Build history of the part. All positions in model axes, mm. A direction names the side the tool comes from. Give positions to 0.01 mm unless a question says otherwise; leave off trailing zeros. Write each loop counter-clockwise with the first axis right and the second up, starting at its lowest first coordinate (ties: lowest second). Pieces come first, ordered by that corner, then holes. Notation, with made-up numbers: M -14,86 L -1,86 A7 cw -1,93 Z; hole C -13.75,88.5 d11. An arc over 180 degrees is marked long. Return JSON: item names as keys, results as strings. Group by question number.
Q1. Pull direction X, two halves, no side cores. Call faces 5 (the flat face through (-2, 2, -12.7)), 6 (the flat face through (-2, -12.7, 0)), 7 (the flat face through (6.35, 19, -10)): +X half, -X half, draft (parallel to the pull), parting line (faces both ways), or undercut.
Q2. Band-saw the part on B-B, the plane y = 9. Give the cut face in (x, z), then the cut area to 3 significant figures.
Q3. Band-saw the part on A-A, the plane y = -23. Give the cut face in (x, z), then the cut area to 3 significant figures.
Q4. Flat gauge pins, fed straight in: pin 1 Ø3 at (y, z) = (-71, -4.5) entering from +X; pin 2 Ø5 at (x, y) = (-9.5, 20.5) entering from -Z; pin 3 Ø5 at (y, z) = (20, 10) entering from +X. Where does each tip first touch, or does it go through?
Q5. Band-saw the part on C-C, the plane x = -17.5. Give the cut face in (y, z), then the cut area to 3 significant figures.
Q6. Tool access for faces 1 (the flat face through (-6.35, 19, -10)), 2 (the flat face through (9, 19, 6.35)), 3 (the flat face through (-12.7, 19, 0)), 4 (the flat face through (9, 19, -6.35)): list every direction of +Z, -Z, +X, -X, +Y, -Y with a clear straight run to the whole face (end or side of a thin tool).
Q7. Wall check: probe 1 along Y at (x, z) = (-132, -6.5); probe 2 along X at (y, z) = (-13, -1.25); probe 3 along X at (y, z) = (15.5, 3.5). Give the ranges that are in metal, low to high.
from build123d import *
from build123d import SkipClean  # not in build123d's __all__

# Parameters (mm, degrees)
F1_DEPTH = 82.5
F0_W     = 12.7
F0_H     = 6.35
F2_DEPTH = 12.7
F0_W_2   = 6.35
F0_H_2   = 12.7
F4_DEPTH = 25.4
F5_DEPTH = 12.7


# Not quite as in the source:
# - after a boolean that leaves OpenCascade's solid faulty, fix() repairs it
# - a feature of the source that left no trace in its solid (it failed there, or was rolled back) is left out
# - a feature names something its author has since deleted; it is built from what else it names


with BuildPart() as f1:
    # F0 (on Front) → F1 (new body)
    with BuildSketch(Plane.XZ):
        with BuildLine():
            Line((-139.7, 0), (-139.7, 12.7))
            ThreePointArc((-139.7, 12.7), (-148.6802561211, 8.9802561211), (-152.4, 0))
            Line((-152.4, 0), (-139.7, 0))
        make_face()
        with BuildLine():
            ThreePointArc((-127, 0), (-130.7197438789, 8.9802561211), (-139.7, 12.7))
            Line((-139.7, 12.7), (-139.7, 0))
            Line((-139.7, 0), (-139.7, -12.7))
            ThreePointArc((-139.7, -12.7), (-130.7197438789, -8.9802561211), (-127, 0))
        make_face()
        with BuildLine():
            Line((-139.7, -12.7), (-139.7, 0))
            Line((-139.7, 0), (-152.4, 0))
            ThreePointArc((-152.4, 0), (-148.6802561211, -8.9802561211), (-139.7, -12.7))
        make_face()
        with BuildLine():
            ThreePointArc((-127, 0), (-130.7197438789, 8.9802561211), (-139.7, 12.7))
            Line((-139.7, 12.7), (-139.7, 0))
            Line((-139.7, 0), (-139.7, -12.7))
            ThreePointArc((-139.7, -12.7), (-130.7197438789, -8.9802561211), (-127, 0))
        make_face()
    extrude(amount=F1_DEPTH)



with BuildPart() as f1b:
    # F0 (on Front) → F1, piece 2 (new body)
    with BuildSketch(Plane.XZ):
        with BuildLine():
            Line((139.7, -12.7), (139.7, 12.7))
            ThreePointArc((139.7, 12.7), (127, 0), (139.7, -12.7))
        make_face()
        with BuildLine():
            ThreePointArc((152.4, 0), (148.6802561211, 8.9802561211), (139.7, 12.7))
            Line((139.7, 12.7), (139.7, -12.7))
            ThreePointArc((139.7, -12.7), (148.6802561211, -8.9802561211), (152.4, 0))
        make_face()
        with BuildLine():
            ThreePointArc((152.4, 0), (148.6802561211, 8.9802561211), (139.7, 12.7))
            Line((139.7, 12.7), (139.7, -12.7))
            ThreePointArc((139.7, -12.7), (148.6802561211, -8.9802561211), (152.4, 0))
        make_face()
    extrude(amount=F1_DEPTH)


with BuildPart() as f1_1:
    add(f1.part, clean=False)

    with SkipClean():  # cleaning this boolean's faces spoils the solid; the shape is the same uncleaned
        add(f1b.part)  # F2 merges F1b
    # F0 (on Front) → F2 (join, symmetric)
    with BuildSketch(Plane.XZ):
        with BuildLine():
            Line((139.7, 12.7), (6.35, 12.7))
            Line((6.35, 12.7), (6.35, 6.35))
            Line((6.35, 6.35), (12.7, 6.35))
            Line((12.7, 6.35), (12.7, -6.35))
            Line((12.7, -6.35), (6.35, -6.35))
            Line((6.35, -6.35), (6.35, -12.7))
            Line((6.35, -12.7), (139.7, -12.7))
            ThreePointArc((139.7, -12.7), (127, 0), (139.7, 12.7))
        make_face()
        with BuildLine():
            Line((139.7, -12.7), (139.7, 12.7))
            ThreePointArc((139.7, 12.7), (127, 0), (139.7, -12.7))
        make_face()
        with BuildLine():
            Line((139.7, -12.7), (139.7, 12.7))
            ThreePointArc((139.7, 12.7), (127, 0), (139.7, -12.7))
        make_face()
        with BuildLine():
            ThreePointArc((152.4, 0), (148.6802561211, 8.9802561211), (139.7, 12.7))
            Line((139.7, 12.7), (139.7, -12.7))
            ThreePointArc((139.7, -12.7), (148.6802561211, -8.9802561211), (152.4, 0))
        make_face()
        with BuildLine():
            Line((-139.7, 0), (-139.7, 12.7))
            ThreePointArc((-139.7, 12.7), (-148.6802561211, 8.9802561211), (-152.4, 0))
            Line((-152.4, 0), (-139.7, 0))
        make_face()
        with BuildLine():
            Line((-139.7, -12.7), (-139.7, 0))
            Line((-139.7, 0), (-152.4, 0))
            ThreePointArc((-152.4, 0), (-148.6802561211, -8.9802561211), (-139.7, -12.7))
        make_face()
        with BuildLine():
            ThreePointArc((-127, 0), (-130.7197438789, 8.9802561211), (-139.7, 12.7))
            Line((-139.7, 12.7), (-139.7, 0))
            Line((-139.7, 0), (-139.7, -12.7))
            ThreePointArc((-139.7, -12.7), (-130.7197438789, -8.9802561211), (-127, 0))
        make_face()
        with BuildLine():
            Line((-6.35, 12.7), (-139.7, 12.7))
            ThreePointArc((-139.7, 12.7), (-130.7197438789, 8.9802561211), (-127, 0))
            ThreePointArc((-127, 0), (-130.7197438789, -8.9802561211), (-139.7, -12.7))
            Line((-139.7, -12.7), (-6.35, -12.7))
            Line((-6.35, -12.7), (-6.35, -6.35))
            Line((-6.35, -6.35), (-12.7, -6.35))
            Line((-12.7, -6.35), (-12.7, 6.35))
            Line((-12.7, 6.35), (-6.35, 6.35))
            Line((-6.35, 6.35), (-6.35, 12.7))
        make_face()
        with Locations((0, 9.525)):
            Rectangle(F0_W, F0_H)
    with SkipClean():  # cleaning this boolean's faces spoils the solid; the shape is the same uncleaned
        extrude(amount=F2_DEPTH, both=True)

    # F0 (on Front) → F4 (join)
    with BuildSketch(Plane.XZ):
        with Locations((-9.525, 0)):
            Rectangle(F0_W_2, F0_H_2)
        Rectangle(F0_W, F0_H_2)
        with Locations((0, 9.525)):
            Rectangle(F0_W, F0_H)
        with Locations((9.525, 0)):
            Rectangle(F0_W_2, F0_H_2)
        with Locations((0, -9.525)):
            Rectangle(F0_W, F0_H)
    extrude(amount=-F4_DEPTH)

    add(f1_1.part.fix(), mode=Mode.REPLACE)

    # F0 (on Front) → F5 (join)
    with BuildSketch(Plane.XZ):
        with Locations((9.525, 0)):
            Rectangle(F0_W_2, F0_H_2)
        with Locations((0, -9.525)):
            Rectangle(F0_W, F0_H)
        with Locations((0, 9.525)):
            Rectangle(F0_W, F0_H)
        with Locations((-9.525, 0)):
            Rectangle(F0_W_2, F0_H_2)
        Rectangle(F0_W, F0_H_2)
    extrude(amount=F5_DEPTH)


solid = f1_1.part
From the geometry:
{
 "1": {"face 5": "draft", "face 6": "undercut", "face 7": "+X half"},
 "2": {"outline": "M -139.7,-12.7 L 139.7,-12.7 A12.7 ccw 139.7,12.7 L -139.7,12.7 A12.7 ccw Z", "area": "7,600 mm^2"},
 "3": {"outline": "C -139.7,0 d25.4; C 139.7,0 d25.4", "area": "1,010 mm^2"},
 "4": {"pin 1": "stops at x = 152.04", "pin 2": "stops at z = -6.35", "pin 3": "stops at x = 6.35"},
 "5": {"outline": "M -12.7,-12.7 L 12.7,-12.7 L 12.7,12.7 L -12.7,12.7 Z", "area": "645 mm^2"},
 "6": {"face 1": "-Z, -X, +Y", "face 2": "+Z, +X, +Y", "face 3": "+Z, -Z, -X, +Y", "face 4": "-Z, +X, +Y"},
 "7": {"probe 1": "y = -82.5 to 12.7", "probe 2": "x = -152.34 to -127.06, 127.06 to 152.34", "probe 3": "x = -12.7 to 12.7"}
}
